Check sheet for the modelled part. Datum: model origin and axes. Units: mm. A direction names the side the tool comes from. Round coordinates to 2 decimals unless told otherwise and drop trailing zeros. Order: outer loops, then holes, each group sorted by start corner. A loop starts at its lowest first (then second) coordinate and runs counter-clockwise, first axis right, second up.
(1) Depth check by flat-ended pin: pin 1 (3 mm diameter, centred on x = 23, z = 3.5, fed in from +Y); pin 2 (4 mm diameter, centred on x = -25, z = 2.5, fed in from +Y); pin 3 (3 mm diameter, centred on x = 0, z = 4, fed in from +Y). Enter the tip coordinate at first touch or a pass-through.
(2) Sectioned sample at A-A, the plane y = 17.5. Enter the section's corners in (x, z).
(3) Thickness scan on probe 1 along X at (y, z) = (-2, 2); probe 2 along X at (y, z) = (5, 2.5); probe 3 along Y at (x, z) = (0, 5.25). Record the ranges inside material, lowest first.
(4) Sectioned sample at C-C, the plane z = 4. Count the separate pieces of the cut face and the enclosed holes in it, and give its area (3 significant figures).
(5) Mould release check, pull along X, two halves, no side actions. Record for faces 1 (the flat face through (3.84, 28.34, 3.45)), 2 (the cylindrical face through (-12.23, -4.98, 3.55)), 3 (the flat face through (-3.726, 30.976, 3.451)): released by +X, released by -X, zero draft, split by the parting line, or undercut.
(6) Tool access check on faces 4 (the flat face through (22.62, -17.494, 3.451)), 5 (the flat face through (12.076, 11.234, 3.549)), 6 (the flat face through (0.44, 39.56, 3.45)). Record the directions out of +Z, -Z, +X, -X, +Y, -Y that give a thin tool (end or side, any length) a straight path to the whole face; none if there is none.
(7) Sectioned sample at B-B, the plane x = 24.5. Enter the section's corners in (y, z), and give its area (3 significant figures).
```python
from build123d import *

# Parameters (mm, degrees)
F0_R       = 11
F1_DEPTH   = 7
F3_DEPTH   = 25
F4_SIZE2   = 11
F4_SIZE    = 6
F4_2_SIZE2 = 11
F4_2_SIZE  = 6
F4_3_SIZE2 = 11
F4_3_SIZE  = 6
F6_DEPTH   = 25


with BuildPart() as f1:
    # F0 (on Top) → F1 (new body)
    with BuildSketch(Plane.XY):
        with BuildLine():
            ThreePointArc((20.0661304609, -4.388266099), (20.4214599699, -2.2069081826), (20.5403619985, 0))
            ThreePointArc((20.5403619985, 0), (16.3588873239, 12.4214844746), (5.5169386953, 19.7855972481))
            ThreePointArc((5.5169386953, 19.7855972481), (-0.3734961981, 20.5369659789), (-6.2327153102, 19.5719117843))
            ThreePointArc((-6.2327153102, 19.5719117843), (-17.9722823534, 9.9450257937), (-19.8932991935, -5.1149895628))
            ThreePointArc((-19.8932991935, -5.1149895628), (-17.5987861554, -10.5919401852), (-13.8334151507, -15.1836456853))
            ThreePointArc((-13.8334151507, -15.1836456853), (0.3734961981, -20.5369659789), (14.3763604982, -14.6706076853))
            ThreePointArc((14.3763604982, -14.6706076853), (17.9722823534, -9.9450257937), (20.0661304609, -4.388266099))
        make_face()
        Circle(F0_R, mode=Mode.SUBTRACT)
        with BuildLine():
            ThreePointArc((-6.2327153102, 19.5719117843), (-0.3734961981, 20.5369659789), (5.5169386953, 19.7855972481))
            Line((5.5169386953, 19.7855972481), (0, 47.9250028729))
            Line((0, 47.9250028729), (-6.2327153102, 19.5719117843))
        make_face()
        with BuildLine():
            Line((41.5042699644, -23.9625014365), (20.0661304609, -4.388266099))
            ThreePointArc((20.0661304609, -4.388266099), (17.9722823534, -9.9450257937), (14.3763604982, -14.6706076853))
            Line((14.3763604982, -14.6706076853), (41.5042699644, -23.9625014365))
        make_face()
        with BuildLine():
            ThreePointArc((-13.8334151507, -15.1836456853), (-17.5987861554, -10.5919401852), (-19.8932991935, -5.1149895628))
            Line((-19.8932991935, -5.1149895628), (-41.5042699644, -23.9625014365))
            Line((-41.5042699644, -23.9625014365), (-13.8334151507, -15.1836456853))
        make_face()
    extrude(amount=F1_DEPTH)

    # F2 (on face) → F3 (cut)
    with BuildSketch(Plane.XY.offset(7)):
        with BuildLine():
            Line((-9.5540666953, 9.1768233106), (-13.7369418517, 12.9794366658))
            ThreePointArc((-13.7369418517, 12.9794366658), (-17.4606316299, -7.0968885961), (-0.7769295863, -18.868837785))
            Line((-0.7769295863, -18.868837785), (-0.8080550469, -13.1635311991))
            ThreePointArc((-0.8080550469, -13.1635311991), (-12.3077837352, -4.7833902956), (-9.5540666953, 9.1768233106))
        make_face()
        with BuildLine():
            ThreePointArc((1.5056530058, -18.8563850914), (18.0599213945, -6.9031052193), (14.1174058688, 13.1313968438))
            Line((14.1174058688, 13.1313968438), (9.9762689865, 9.2833716066))
            ThreePointArc((9.9762689865, 9.2833716066), (12.882138258, -4.6459659672), (1.4745275451, -13.1510785055))
            Line((1.4745275451, -13.1510785055), (1.5056530058, -18.8563850914))
        make_face()
        with BuildLine():
            ThreePointArc((13.2514961216, 14.0726582684), (0.156741732, 19.1941948225), (-12.8813534975, 13.9300897717))
            Line((-12.8813534975, 13.9300897717), (-8.888608776, 10.2225420997))
            ThreePointArc((-8.888608776, 10.2225420997), (0.1864346526, 13.7514732817), (9.2994411209, 10.3217675178))
            Line((9.2994411209, 10.3217675178), (13.2514961216, 14.0726582684))
        make_face()
    extrude(amount=-F3_DEPTH, mode=Mode.SUBTRACT)

    # F4
    f4_edges = [f1.edges().sort_by_distance(p)[0] for p in [
        (-41.50427, -23.962501, 3.5),
    ]]
    f4_side = f1.faces().sort_by_distance((-27.668843, -19.573074, 3.5))[0]
    chamfer(f4_edges, length=F4_SIZE, length2=F4_SIZE2, reference=f4_side)

    # F4#2
    f4_2_edges = [f1.edges().sort_by_distance(p)[0] for p in [
        (0, 47.925003, 3.5),
    ]]
    f4_2_side = f1.faces().sort_by_distance((-3.116358, 33.748457, 3.5))[0]
    chamfer(f4_2_edges, length=F4_2_SIZE, length2=F4_2_SIZE2, reference=f4_2_side)

    # F4#3
    f4_3_edges = [f1.edges().sort_by_distance(p)[0] for p in [
        (41.50427, -23.962501, 3.5),
    ]]
    f4_3_side = f1.faces().sort_by_distance((30.7852, -14.175384, 3.5))[0]
    chamfer(f4_3_edges, length=F4_3_SIZE, length2=F4_3_SIZE2, reference=f4_3_side)

    # F5 (on face) → F6 (cut)
    with BuildSketch(Plane.XY.offset(7)):
        with BuildLine():
            ThreePointArc((-4.1133450785, 21.7607795339), (-0.3226835167, 22.146741457), (3.4775948856, 21.8711226117))
            Line((3.4775948856, 21.8711226117), (0.6102930376, 36.4959307173))
            Line((0.6102930376, 36.4959307173), (-0.515505202, 38.1276239452))
            Line((-0.515505202, 38.1276239452), (-4.1133450785, 21.7607795339))
        make_face()
        with BuildLine():
            Line((-20.6797452338, -7.9238757909), (-31.9115496548, -17.7194360843))
            Line((-31.9115496548, -17.7194360843), (-32.7617383215, -19.5102525733))
            Line((-32.7617383215, -19.5102525733), (-16.7887153433, -14.4426510995))
            ThreePointArc((-16.7887153433, -14.4426510995), (-19.0182989544, -11.3528228513), (-20.6797452338, -7.9238757909))
        make_face()
        with BuildLine():
            Line((17.2021503482, -13.9472468209), (31.3012566171, -18.776494633))
            Line((31.3012566171, -18.776494633), (33.2772435235, -18.6173713719))
            Line((33.2772435235, -18.6173713719), (20.9020604218, -7.3181284344))
            ThreePointArc((20.9020604218, -7.3181284344), (19.3409824711, -10.7939186057), (17.2021503482, -13.9472468209))
        make_face()
    extrude(amount=-F6_DEPTH, mode=Mode.SUBTRACT)


solid = f1.part
```
Derived:
1. pin 1: stops at y = -5.7
1. pin 2: stops at y = -7.82
1. pin 3: stops at y = 42.06
2. outline: (-10.75, 0) - (-7.59, 0) - (-7.59, 7) - (-10.75, 7) - close; (8.11, 0) - (10.75, 0) - (10.75, 7) - (8.11, 7) - close
3. probe 1: x = -20.44 to -18.75, -13.06 to -10.82, 10.82 to 13.58, 19.27 to 20.44
3. probe 2: x = -19.92 to -18.19, -12.25 to -9.8, 9.8 to 12.78, 18.72 to 19.92
3. probe 3: y = -20.54 to -11, 11 to 13.75, 19.19 to 22.15, 37.38 to 40.2
4. separate pieces: 1
4. enclosed holes: 7
4. area: 639 mm2
5. face 1: released by +X
5. face 2: undercut
5. face 3: released by -X
6. face 4: +Z, -Z, -Y
6. face 5: +Z, -Z
6. face 6: +Z, -Z, +X, +Y
7. outline: (-18.14, 0) - (-16.45, 0) - (-16.45, 7) - (-18.14, 7) - close; (-10.6, 0) - (-8.44, 0) - (-8.44, 7) - (-10.6, 7) - close
7. area: 27.0 mm2
